Part model, mm, in its own coordinate system. A direction names the side the tool comes from. Round coordinates to 2 decimals unless told otherwise and drop trailing zeros. Loops run counter-clockwise (first coordinate to the right, second up) from the corner with the lowest first, then second, coordinate; pieces in that order, holes last.
from build123d import *

# Parameters (mm, degrees)
SKETCH1_W           = 29
SKETCH1_H           = 44
SKETCH1_W_2         = 18
SKETCH1_H_2         = 33
BOSS_EXTRUDE1_DEPTH = 5.5
SKETCH2_R           = 2.6
SKETCH2_R_2         = 2
SKETCH2_R_3         = 1.05
BOSS_EXTRUDE2_DEPTH = 2.9
SKETCH2_4_R         = 2
SKETCH2_4_R_2       = 1.05
CUT_EXTRUDE1_DEPTH  = 1.4
BOSS_EXTRUDE4_START = -11.6
BOSS_EXTRUDE4_DEPTH = 23.2
FILLET1_R           = 2


with BuildPart() as part:
    # Sketch1 → Boss-Extrude1 (new body)
    with BuildSketch(Plane(origin=(0, 0, 0), x_dir=(1, 0, 0), z_dir=(0, 1, 0))):
        Rectangle(SKETCH1_W, SKETCH1_H)
        Rectangle(SKETCH1_W_2, SKETCH1_H_2, mode=Mode.SUBTRACT)
    extrude(amount=BOSS_EXTRUDE1_DEPTH)

    # Sketch2 → Boss-Extrude2 (add)
    # profile 1 of 6: a face of its own
    with BuildSketch(Plane(origin=(14.5, 0, 0), x_dir=(0, 0, -1), z_dir=(1, 0, 0))):
        with BuildLine():
            Line((-17, -3), (-17, 0))
            Line((-17, 0), (-22, 0))
            Line((-22, 0), (-22, 5.5))
            Line((-22, 5.5), (-25.4, 5.5))
            ThreePointArc((-25.4, 5.5), (-33.248885271, 2.248885271), (-36.5, -5.6))
            Line((-36.5, -5.6), (-19.6, -5.6))
            ThreePointArc((-19.6, -5.6), (-21.438477631, -1.161522369), (-17, -3))
        make_face()
    # profile 2 of 6: a face of its own
    with BuildSketch(Plane(origin=(14.5, 0, 0), x_dir=(0, 0, -1), z_dir=(1, 0, 0))):
        with Locations((-19.6, -3)):
            Circle(SKETCH2_R)
        with Locations((-19.6, -3)):
            Circle(SKETCH2_R_2, mode=Mode.SUBTRACT)
    # profile 3 of 6: a face of its own
    with BuildSketch(Plane(origin=(14.5, 0, 0), x_dir=(0, 0, -1), z_dir=(1, 0, 0))):
        with Locations((19.4, -3)):
            Circle(SKETCH2_R)
        with Locations((19.4, -3)):
            Circle(SKETCH2_R_2, mode=Mode.SUBTRACT)
    # profile 4 of 6: a face of its own
    with BuildSketch(Plane(origin=(14.5, 0, 0), x_dir=(0, 0, -1), z_dir=(1, 0, 0))):
        with BuildLine():
            Line((22, -3), (22, 0))
            Line((22, 0), (16.8, 0))
            Line((16.8, 0), (16.8, -3))
            ThreePointArc((16.8, -3), (19.4, -0.4), (22, -3))
        make_face()
    # profile 5 of 6: a face of its own
    with BuildSketch(Plane(origin=(14.5, 0, 0), x_dir=(0, 0, -1), z_dir=(1, 0, 0))):
        with Locations((-19.6, -3)):
            Circle(SKETCH2_R_2)
        with Locations((-19.6, -3)):
            Circle(SKETCH2_R_3, mode=Mode.SUBTRACT)
    # profile 6 of 6: a face of its own
    with BuildSketch(Plane(origin=(14.5, 0, 0), x_dir=(0, 0, -1), z_dir=(1, 0, 0))):
        with Locations((19.4, -3)):
            Circle(SKETCH2_R_2)
        with Locations((19.4, -3)):
            Circle(SKETCH2_R_3, mode=Mode.SUBTRACT)
    boss_extrude2 = extrude(amount=-BOSS_EXTRUDE2_DEPTH)

    # Sketch2_4 → Cut-Extrude1 (cut)
    # profile 1 of 2: a face of its own
    with BuildSketch(Plane(origin=(14.5, 0, 0), x_dir=(0, 0, -1), z_dir=(1, 0, 0))):
        with Locations((-19.6, -3)):
            Circle(SKETCH2_4_R)
        with Locations((-19.6, -3)):
            Circle(SKETCH2_4_R_2, mode=Mode.SUBTRACT)
    # profile 2 of 2: a face of its own
    with BuildSketch(Plane(origin=(14.5, 0, 0), x_dir=(0, 0, -1), z_dir=(1, 0, 0))):
        with Locations((19.4, -3)):
            Circle(SKETCH2_4_R)
        with Locations((19.4, -3)):
            Circle(SKETCH2_4_R_2, mode=Mode.SUBTRACT)
    cut_extrude1 = extrude(amount=-CUT_EXTRUDE1_DEPTH, mode=Mode.SUBTRACT)

    # Mirror1: Boss-Extrude2, Cut-Extrude1 across plane
    add(boss_extrude2.mirror(Plane(origin=(0, 0, 0), x_dir=(0, 0, 1), z_dir=(1, 0, 0))))
    add(cut_extrude1.mirror(Plane(origin=(0, 0, 0), x_dir=(0, 0, 1), z_dir=(1, 0, 0))), mode=Mode.SUBTRACT)

    # Sketch3 → Boss-Extrude4 (add)
    with BuildSketch(Plane(origin=(0, 0, 0), x_dir=(0, 0, -1), z_dir=(1, 0, 0)).offset(BOSS_EXTRUDE4_START)):
        with BuildLine():
            Line((-31.5, 0), (-22, 0))
            Line((-22, 0), (-22, 5.5))
            Line((-22, 5.5), (-25.4, 5.5))
            ThreePointArc((-25.4, 5.5), (-29.920514853, 4.537797861), (-33.657309154, 1.818008192))
            ThreePointArc((-33.657309154, 1.818008192), (-37.265361906, -0.468563976), (-41.536346157, -0.540330832))
            ThreePointArc((-41.536346157, -0.540330832), (-55.132701751, 0.845458827), (-68.5, -2))
            Line((-68.5, -2), (-68.5, -8.5))
            ThreePointArc((-68.5, -8.5), (-52.75, -5.090094938), (-37, -8.5))
            ThreePointArc((-37, -8.5), (-34.608858311, -6.369406651), (-31.5, -5.6))
            Line((-31.5, -5.6), (-31.5, 0))
        make_face()
    extrude(amount=BOSS_EXTRUDE4_DEPTH)

    # Fillet1
    fillet1_edges = [part.edges().sort_by_distance(p)[0] for p in [
        (0, 5.5, -22),
    ]]
    fillet(fillet1_edges, radius=FILLET1_R)


solid = part.part
1) Drop flat-ended pins along their axis: pin 1 Ø3 at (x, y) = (-13.5, -2) entering from +Z; pin 2 Ø4.5 at (y, z) = (-3, -19.4) entering from +X; pin 3 Ø2 at (x, y) = (2, -5.5) entering from -Z; pin 4 Ø1.5 at (x, z) = (-7, 51) entering from -Y. Give the stop position or say it passes through.
Values:
pin 1: stops at z = 36.3
pin 2: stops at x = 14.5
pin 3: stops at z = 31.5
pin 4: stops at y = -5.17
2) Slice it at A-A, the plane z = -6.5. Give the cut face in (x, y).
Values:
outline: (-14.5, 0) - (-9, 0) - (-9, 5.5) - (-14.5, 5.5) - close; (9, 0) - (14.5, 0) - (14.5, 5.5) - (9, 5.5) - close
3) Mould opens along Y. For faces 1 (the face through (-13.81, -2.399, 17.692)), 2 (the face through (-13, -5.6, 28)), 3 (the face through (-11.6, -3, 24)), 4 (the face through (-13.1, -3.9, -20.3)) say: released by +Y, released by -Y, zero draft, split by the parting line, or undercut.
Values:
face 1: undercut
face 2: released by -Y
face 3: zero draft
face 4: undercut
4) Slice it at B-B, the plane x = -6. Give the cut face in (y, z), then the cut area to 3 significant figures.
Values:
outline: (-8.5, 37) arc R6.67 cw to (-5.6, 31.5) - (0, 31.5) - (0, 16.5) - (5.5, 16.5) - (5.5, 25.4) arc R11.1 ccw to (1.82, 33.66) arc R7.89 cw to (-0.54, 41.54) arc R44.08 ccw to (-2, 68.5) - (-8.5, 68.5) arc R38.08 cw to start; (0, -22) - (3.5, -22) arc R2 ccw to (5.5, -20) - (5.5, -16.5) - (0, -16.5) - close
area: 348 mm2
5) Slice it at C-C, the plane z = 23.5. Give the cut face in (x, y), then the cut area to 3 significant figures.
Values:
outline: (-14.5, -5.6) - (-11.6, -5.6) - (-11.6, 0) - (11.6, 0) - (11.6, -5.6) - (14.5, -5.6) - (14.5, 5.5) - (-14.5, 5.5) - close
area: 192 mm2
6) Tool access for faces 5 (the face through (9, 3, 0)), 6 (the face through (13.07, -4.859, 17.782)), 7 (the face through (-13.1, -3.9, 18.7)), 8 (the face through (13.1, -3.9, 18.7)): list every direction of +Z, -Z, +X, -X, +Y, -Y with a clear straight run to the whole face (end or side of a thin tool).
Values:
face 5: +Y, -Y
face 6: +X, -X, -Y
face 7: -X
face 8: +X
7) Slice it at D-D, the plane y = 4.5. Give the cut face in (x, z), then the cut area to 3 significant figures.
Values:
outline: (-14.5, -21.73) - (14.5, -21.73) - (14.5, 30) - (-14.5, 30) - close; hole (-9, -16.5) - (9, -16.5) - (9, 16.5) - (-9, 16.5) - close
area: 906 mm2
8) Wall check: line 1 along X through (y, z) = (3.5, -15); line 2 along Y through (x, z) = (12.6, -19.4); line 3 along Z through (x, y) = (3.5, -4.75). Give the ranges that are in metal, low to high.
Values:
line 1: x = -14.5 to -9, 9 to 14.5
line 2: y = -5.6 to -4.05, -1.95 to 5.5
line 3: z = 31.5 to 68.5
